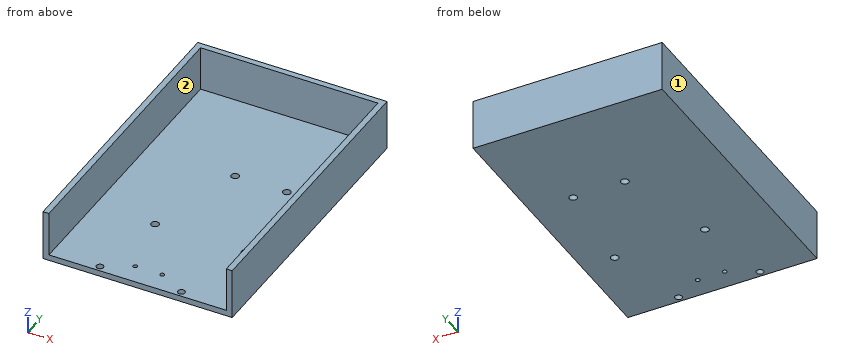
from build123d import *

# Parameters (mm, degrees)
F0_W     = 101.6
F0_H     = 152.4
F1_DEPTH = 3.175
F2_W     = 3.175
F2_H     = 152.4
F3_DEPTH = 24.13
F4_W     = 101.6
F4_H     = 27.305
F5_DEPTH = 3.175
F6_R     = 1.875
F6_R_2   = 1.175
F6_R_3   = 2.1
F6_R_4   = 1.625
F7_DEPTH = 3.175


with BuildPart() as f1:
    # F0 (on Top) → F1 (new body)
    with BuildSketch(Plane.XY):
        with Locations((0, 1.825321)):
            Rectangle(F0_W, F0_H)
    extrude(amount=F1_DEPTH)

    # F2 (on face) → F3 (join)
    with BuildSketch(Plane.XY.offset(3.175)):
        with Locations((49.2125, 1.825321)):
            Rectangle(F2_W, F2_H)
        with Locations((-49.2125, 1.825321)):
            Rectangle(F2_W, F2_H)
    extrude(amount=F3_DEPTH)

    # F4 (on face) → F5 (join)
    with BuildSketch(Plane(origin=(0, 78.025321, 0), x_dir=(-1, 0, 0), z_dir=(0, 1, 0))):
        with Locations((0, 13.6525)):
            Rectangle(F4_W, F4_H)
    extrude(amount=F5_DEPTH)

    # F6 (on face) → F7 (cut, through all)
    with BuildSketch(Plane.XY.offset(3.175)):
        with Locations((-21.875, -71.249679)):
            Circle(F6_R)
        with Locations((21.875, -71.249679)):
            Circle(F6_R)
        with Locations((-7.25, -63.199679)):
            Circle(F6_R_2)
        with Locations((7.25, -63.199679)):
            Circle(F6_R_2)
        with Locations((-15.060561, -28.659923)):
            Circle(F6_R_3)
        with Locations((-15.060561, -28.659923)):
            Circle(F6_R_4, mode=Mode.SUBTRACT)
        with Locations((27.789439, 23.580077)):
            Circle(F6_R_3)
        with Locations((27.789439, 23.580077)):
            Circle(F6_R_4, mode=Mode.SUBTRACT)
        with Locations((0.039439, 23.580077)):
            Circle(F6_R_3)
        with Locations((0.039439, 23.580077)):
            Circle(F6_R_4, mode=Mode.SUBTRACT)
        with Locations((33.419439, -28.659923)):
            Circle(F6_R_3)
        with Locations((33.419439, -28.659923)):
            Circle(F6_R_4, mode=Mode.SUBTRACT)
        with Locations((27.789439, 23.580077)):
            Circle(F6_R_4)
        with Locations((33.419439, -28.659923)):
            Circle(F6_R_4)
        with Locations((-15.060561, -28.659923)):
            Circle(F6_R_4)
        with Locations((0.039439, 23.580077)):
            Circle(F6_R_4)
    extrude(amount=-F7_DEPTH, mode=Mode.SUBTRACT)


solid = f1.part
The model under review builds one solid part; all positions refer to its coordinate system, in mm. Face numbers are marked on the shaded views. A direction names the side the tool comes from. Coordinates: 2 decimals unless noted, no trailing zeros. Write each loop counter-clockwise with the first axis right and the second up, starting at its lowest first coordinate (ties: lowest second). Pieces come first, ordered by that corner, then holes. Notation, with made-up numbers: (-37.5, 6.25) - (0.5, 6.25) arc R20 cw to (0.5, 40.25) - close; hole circle Ø2 at (60, 70.25). An arc over 180 degrees is marked (long way). Answer as a JSON object with one key per item and string values. Group by question number.
1. To check wall thickness, follow probe 1 along X at (y, z) = (25, 22.5) (3 decimals); probe 2 along Y at (x, z) = (-7.25, 2.35); probe 3 along Z at (x, y) = (41.5, -33) (3 decimals). State the ranges of each line that lie inside material, in increasing order.
2. Clearance check with flat-ended pins moving along their axes: pin 1 Ø4 at (x, y) = (7.25, -63.2) entering from +Z (3 decimals); pin 2 Ø12 at (x, z) = (-5.5, 18.5) entering from -Y. State where each tip first meets the part, or that it passes through.
3. Add section B-B (x = 4.5). Give the boundary of the cut face in (y, z) (3 decimals), plus the area to 3 significant figures.
4. Add section A-A (z = 12.75). Give the boundary of the cut face in (x, y) (3 decimals).
5. Machinability: for the marked faces 1 and 2, which of the approach directions +Z, -Z, +X, -X, +Y, -Y give a long, thin tool a straight path to every point of the face, cutting with its end or side? Answer none if there is none.
6. Add section C-C (y = -23). Give the boundary of the cut face in (x, z) (3 decimals).
Findings:
{
 "1": {"probe 1": "-50.8 to -47.625, 47.625 to 50.8", "probe 2": "-74.37 to -64.37, -62.02 to 81.2", "probe 3": "0 to 3.175"},
 "2": {"pin 1": "z = 3.175", "pin 2": "y = 78.03"},
 "3": {"outline": "(-74.375, 0) - (81.2, 0) - (81.2, 27.305) - (78.025, 27.305) - (78.025, 3.175) - (-74.375, 3.175) - close", "area": "571 mm²"},
 "4": {"outline": "(-50.8, -74.375) - (-47.625, -74.375) - (-47.625, 78.025) - (47.625, 78.025) - (47.625, -74.375) - (50.8, -74.375) - (50.8, 81.2) - (-50.8, 81.2) - close"},
 "5": {"face 1": "+Z, -Z, -X, +Y, -Y", "face 2": "+Z, -Y"},
 "6": {"outline": "(-50.8, 0) - (50.8, 0) - (50.8, 27.305) - (47.625, 27.305) - (47.625, 3.175) - (-47.625, 3.175) - (-47.625, 27.305) - (-50.8, 27.305) - close"}
}
